Verification items for the finished model (mm, model axes). Round coordinates to 2 decimals unless told otherwise and drop trailing zeros. Order: outer loops, then holes, each group sorted by start corner. A loop starts at its lowest first (then second) coordinate and runs counter-clockwise, first axis right, second up. Notation, with made-up numbers: M -10.75,41.25 L 23.25,41.25 A14 ccw 23.25,59.25 Z; hole C 27,60.25 d5. An arc over 180 degrees is marked long. Answer as a JSON object with one key per item and string values. Group by question number.
```python
from build123d import *

# Parameters (mm, degrees)
SKETCH1_W           = 117.475
SKETCH1_H           = 84.668868
SKETCH1_R           = 2.6289
SKETCH1_R_2         = 2.667
BOSS_EXTRUDE1_DEPTH = 6.35
SKETCH2_R           = 2.6289
CUT_EXTRUDE1_DEPTH  = 7.35


with BuildPart() as part:
    # Sketch1 → Boss-Extrude1 (new body)
    with BuildSketch(Plane(origin=(0, 0, 0), x_dir=(1, 0, 0), z_dir=(0, 1, 0))):
        with Locations((58.7375, 42.334434)):
            Rectangle(SKETCH1_W, SKETCH1_H)
        with Locations((7.9375, 7.9375)):
            Circle(SKETCH1_R, mode=Mode.SUBTRACT)
        with Locations((109.5375, 7.9375)):
            Circle(SKETCH1_R, mode=Mode.SUBTRACT)
        with Locations((7.9375, 76.731368)):
            Circle(SKETCH1_R_2, mode=Mode.SUBTRACT)
        with Locations((109.5375, 76.731368)):
            Circle(SKETCH1_R_2, mode=Mode.SUBTRACT)
    extrude(amount=BOSS_EXTRUDE1_DEPTH)

    # Sketch2 → Cut-Extrude1 (cut, through all)
    with BuildSketch(Plane(origin=(0, 6.35, 0), x_dir=(1, 0, 0), z_dir=(0, 1, 0))):
        with Locations((109.5375, 32.256790414)):
            Circle(SKETCH2_R)
        with Locations((109.5375, 57.656790414)):
            Circle(SKETCH2_R)
        with Locations((65.0875, 57.656790414)):
            Circle(SKETCH2_R)
        with Locations((65.0875, 32.256790414)):
            Circle(SKETCH2_R)
    extrude(amount=-CUT_EXTRUDE1_DEPTH, mode=Mode.SUBTRACT)


solid = part.part
```
Q1. Cross-section at B-B, the plane y = 4.25. Give the number of separate pieces and of enclosed holes in the cut face, then the cut area to 3 significant figures.
Q2. Cross-section at A-A, the plane z = -59. Record the cut outline in (x, y) (3 decimals), then the cut area to 3 significant figures.
Q3. Thickness scan on line 1 (Z direction, x = 109, y = 4.5); line 2 (X direction, y = 2, z = -34) (3 decimals); line 3 (X direction, y = 3, z = -6) (3 decimals). Record the ranges inside material, lowest first. Write a range as from..to.
Q4. Release check for a two-part mould opening along X. For faces 1 (the face through (107.6, 3.219, -34.034)), 2 (the face through (0, 3, -42)), 3 (the face through (58, 3, 0)), 4 (the face through (117.475, 3, -42)) record: released by +X, released by -X, zero draft, split by the parting line, or undercut.
Conclusion:
{
 "1": {"separate pieces": "1", "enclosed holes": "8", "area": "9,770 mm2"},
 "2": {"outline": "M 0,0 L 62.828,0 L 62.828,6.35 L 0,6.35 Z; M 67.347,0 L 107.278,0 L 107.278,6.35 L 67.347,6.35 Z; M 111.797,0 L 117.475,0 L 117.475,6.35 L 111.797,6.35 Z", "area": "689 mm2"},
 "3": {"line 1": "-84.67..-79.34, -74.12..-60.23, -55.08..-34.83, -29.68..-10.51, -5.36..0", "line 2": "0..63.12, 67.055..107.57, 111.505..117.475", "line 3": "0..6.161, 9.714..107.761, 111.314..117.475"},
 "4": {"face 1": "undercut", "face 2": "released by -X", "face 3": "zero draft", "face 4": "released by +X"}
}
